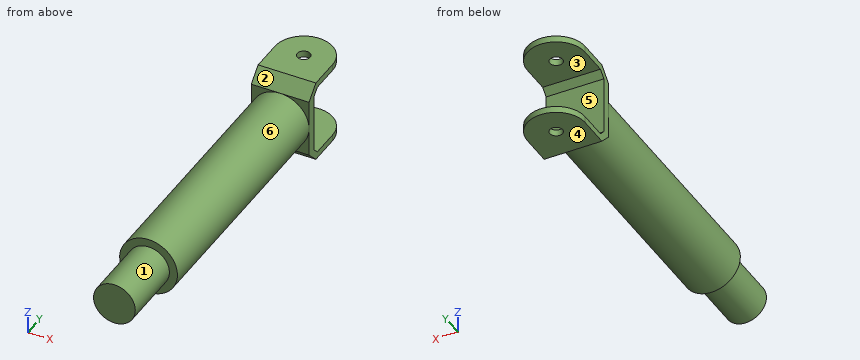
```python
from build123d import *

# Parameters (mm, degrees)
SKETCH1_R               = 32.5
BOSS_EXTRUDE1_DEPTH     = 100
SKETCH2_R               = 45
BOSS_EXTRUDE2_DEPTH     = 400
BOSS_EXTRUDE3_DEPTH     = 45
CUT_EXTRUDE2_DEPTH      = 616.568842616
CUT_EXTRUDE2_DEPTH_BACK = 616.568842616
SKETCH7_R               = 10


with BuildPart() as part:
    # Sketch1 → Boss-Extrude1 (new body)
    with BuildSketch(Plane(origin=(0, 0, 0), x_dir=(1, 0, 0), z_dir=(0, 1, 0))):
        with Locations(Location((0, 0, 0), (0, 0, 270))):
            Circle(SKETCH1_R)
    extrude(amount=BOSS_EXTRUDE1_DEPTH)

    # Sketch2 → Boss-Extrude2 (add)
    with BuildSketch(Plane(origin=(0, 100, 0), x_dir=(1, 0, 0), z_dir=(0, 1, 0))):
        with Locations(Location((0, 0, 0), (0, 0, 270))):
            Circle(SKETCH2_R)
    extrude(amount=BOSS_EXTRUDE2_DEPTH)

    # Sketch6 → Boss-Extrude3 (add, symmetric)
    with BuildSketch(Plane(origin=(0, 0, 0), x_dir=(0, 0, -1), z_dir=(1, 0, 0))):
        Polygon((-45, 500), (-55, 510), (-55, 600), (-65, 600), (-65, 505.857864376), (-45, 485.857864376), (45, 485.857864376), (65, 505.857864376), (65, 600), (55, 600), (55, 510), (45, 500), align=None)
    extrude(amount=BOSS_EXTRUDE3_DEPTH, both=True)

    # Sketch7 → Cut-Extrude2 (cut, two sides: drawn at the far end of the back side and taken through both)
    with BuildSketch(Plane.XY.offset(65).offset(-CUT_EXTRUDE2_DEPTH_BACK)):
        with Locations((0, 555)):
            Circle(SKETCH7_R)
        with BuildLine():
            Line((-45, 555), (-45, 605))
            Line((-45, 605), (45, 605))
            Line((45, 605), (45, 555))
            ThreePointArc((45, 555), (0, 600), (-45, 555))
        make_face()
    extrude(amount=CUT_EXTRUDE2_DEPTH + CUT_EXTRUDE2_DEPTH_BACK, mode=Mode.SUBTRACT)


solid = part.part
```
Could you check a few things on this model? Use its own coordinates, in mm. Face numbers are marked on the shaded views. A direction names the side the tool comes from. Give positions to 0.01 mm unless a question says otherwise; leave off trailing zeros. Loops run counter-clockwise (first coordinate to the right, second up) from the corner with the lowest first, then second, coordinate; pieces in that order, holes last. Notation, with made-up numbers: (75.5, -38.5) - (122.5, -38.5) arc R25 ccw to (122.5, -19.5) - close; hole circle Ø8 at (19.5, -13.75). An arc over 180 degrees is marked (long way). Answer in a Markdown table with one row per item. Add a question column.
Q1. For pin 1 (8 mm diameter, centred on x = -31, z = -21.5, fed in from -Y); pin 2 (1.5 mm diameter, centred on x = -15.5, z = 12.5, fed in from +Y); pin 3 (2 mm diameter, centred on y = 481.5, z = 4, fed in from +X); pin 4 (18 mm diameter, centred on x = 0, y = 555, fed in from -Z), each with a flat end and sliding along its axis, tell me the tip position at first contact or that it passes through.
Q2. If we section it at A-A (x = -26): List the corners of the cut face in (y, z) for me.
Q3. Please list where these lines run through material, in increasing order: L1, parallel to X at y = 555, z = 60.5; L2, parallel to Y at x = 0, z = 59.25; L3, parallel to Z at x = 6.5, y = 571.5. Write a range as from..to.
Q4. If we section it at D-D (x = 20): List the corners of the cut face in (y, z) for me.
Q5. If we section it at C-C (y = 397.5): List the corners of the cut face in (x, z) for me.
Q6. Which directions (+Z, -Z, +X, -X, +Y, -Y) give clear straight access to the entire face, cutting with the end or side of a thin tool? Please do the marked faces 4, 5 and 6.
Q7. If we section it at B-B (z = 7.5): List the corners of the cut face in (x, y) for me, plus the area to 3 significant figures.
Q8. We'd pull the mould along Z, two halves only. Please class the marked faces 1, 2 and 3: +Z half, -Z half, draft (parallel to the pull), parting line (faces both ways), or undercut.
The answers:
| question | item | result |
|---|---|---|
| 1 | pin 1 | stops at y = 100 |
| 1 | pin 2 | stops at y = 500 |
| 1 | pin 3 | stops at x = 44.9 |
| 1 | pin 4 | passes through |
| 2 | outline | (0, -19.5) - (100, -19.5) - (100, -36.73) - (485.86, -36.73) - (485.86, -45) - (505.86, -65) - (591.73, -65) - (591.73, -55) - (510, -55) - (500, -45) - (500, 45) - (510, 55) - (591.73, 55) - (591.73, 65) - (505.86, 65) - (485.86, 45) - (485.86, 36.73) - (100, 36.73) - (100, 19.5) - (0, 19.5) - close |
| 3 | L1 | x = -45..-10, 10..45 |
| 3 | L2 | y = 500.11..545, 565..600 |
| 3 | L3 | z = -65..-55, 55..65 |
| 4 | outline | (0, -25.62) - (100, -25.62) - (100, -40.31) - (485.86, -40.31) - (485.86, -45) - (505.86, -65) - (595.31, -65) - (595.31, -55) - (510, -55) - (500, -45) - (500, 45) - (510, 55) - (595.31, 55) - (595.31, 65) - (505.86, 65) - (485.86, 45) - (485.86, 40.31) - (100, 40.31) - (100, 25.62) - (0, 25.62) - close |
| 5 | outline | circle Ø90 at (0, 0) |
| 6 | face 4 | -Z, +X, -X, +Y, -Y |
| 6 | face 5 | +X, -X, +Y |
| 6 | face 6 | -Y |
| 7 | outline | (-45, 485.86) - (-44.37, 485.86) - (-44.37, 100) - (-31.62, 100) - (-31.62, 0) - (31.62, 0) - (31.62, 100) - (44.37, 100) - (44.37, 485.86) - (45, 485.86) - (45, 500) - (-45, 500) - close |
| 7 | area | 41,800 mm^2 |
| 8 | face 1 | parting line |
| 8 | face 2 | +Z half |
| 8 | face 3 | undercut |
